Study the drawing (mm; zero at the part's minimum x, y, z) and answer. A direction names the side the tool comes from. Give positions to 0.01 mm unless a question says otherwise; leave off trailing zeros. Order: outer loops, then holes, each group sorted by start corner. A loop starts at its lowest first (then second) coordinate and runs counter-clockwise, first axis right, second up. Notation, with made-up numbers: (-26.75, 6) - (23.25, 6) arc R14 cw to (23.25, 12) - close; hole circle Ø8 at (46, 20.5). An arc over 180 degrees is marked (long way). Use CSV: the item, a comma, the result in double quotes.
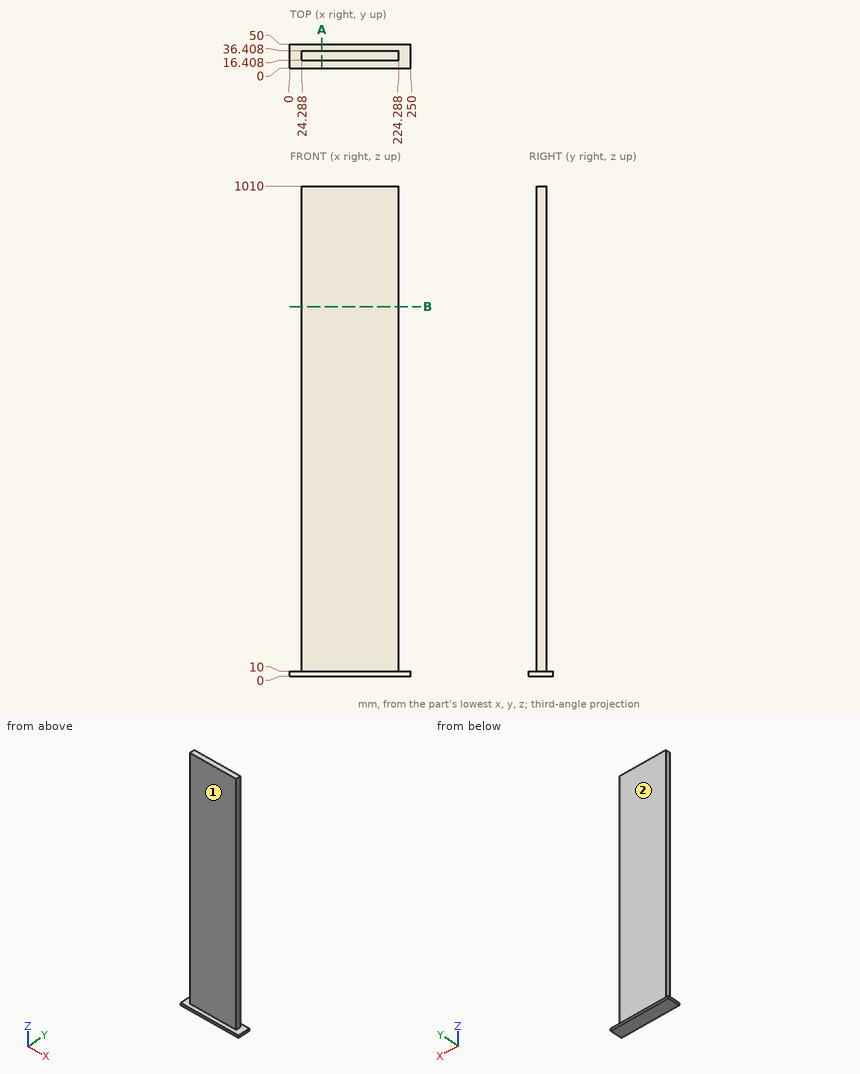
Item 1: Each of these flat-tipped pins is pushed along its axis until it touches: pin 1 (2 mm diameter, centred on x = 88, y = 16.5, fed in from -Z); pin 2 (10 mm diameter, centred on y = 22.5, z = 577.5, fed in from +X); pin 3 (22 mm diameter, centred on y = 23.5, z = 523.5, fed in from -X); pin 4 (1 mm diameter, centred on x = 58.5, z = 364.5, fed in from -Y). Where does it stop, or does it pass through?
Taken from the geometry:
pin 1,"z = 0"
pin 2,"x = 224.29"
pin 3,"x = 24.29"
pin 4,"y = 16.41"
Item 2: The part is cut by section B-B (z = 762). Give the vertices of the cut face in (x, y), and give its area (3 significant figures).
Taken from the geometry:
outline,"(24.29, 16.41) - (224.29, 16.41) - (224.29, 36.41) - (24.29, 36.41) - close"
area,"4,000 mm^2"
Item 3: Which of the six approach directions +Z, -Z, +X, -X, +Y, -Y give full straight-line access (tool end or side, diameter ignored) to the marked faces 1 and 2?
Taken from the geometry:
face 1,"+Z, +X, -X, -Y"
face 2,"+Z, +X, -X, +Y"
Item 4: Find the intervals of material crossed by line 1 along X through (y, z) = (27, 446); line 2 along Y through (x, z) = (214, 893.5); line 3 along Z through (x, y) = (20.5, 41), in increasing order.
Taken from the geometry:
line 1,"24.29 to 224.29"
line 2,"16.41 to 36.41"
line 3,"0 to 10"
Item 5: The part is cut by section A-A (x = 66). Give the vertices of the cut face in (y, z).
Taken from the geometry:
outline,"(0, 0) - (50, 0) - (50, 10) - (36.41, 10) - (36.41, 1010) - (16.41, 1010) - (16.41, 10) - (0, 10) - close"
